CAD build for the part. Positions are in the model's coordinates, mm. Face numbers are marked on the shaded views. A direction names the side the tool comes from. Give positions to 0.01 mm unless a question says otherwise; leave off trailing zeros. Loops run counter-clockwise (first coordinate to the right, second up) from the corner with the lowest first, then second, coordinate; pieces in that order, holes last.
Item 1: Probe probe 1 along Y at (x, z) = (0, 6); probe 2 along Y at (x, z) = (0, -6.25); probe 3 along Y at (x, z) = (-18, 3.5). List the from-to ranges inside material, lowest first.
Item 2: Saw through at B-B on z = -10. Give the cut face in (x, y).
Item 3: Drop flat-ended pins along their axis: P1, Ø1.3, axis at y = 19, z = 0, coming from the +X side; P2, Ø3.5, axis at y = -18.5, z = 4.5, coming from the -X side; P3, Ø5, axis at x = 14, y = -3, coming from the -Z side; P4, Ø6, axis at x = -0.5, z = 5, coming from the +Y side. Give the stop position or say it passes through.
Item 4: Mould opens along X. For the marked faces 6, 7, 8 and 9 say: released by +X, released by -X, zero draft, split by the parting line, or undercut.
Item 5: Which spindle directions (+Z, -Z, +X, -X, +Y, -Y) get a long thin tool onto all of the face, cutting with end or side? Do the marked faces 1, 2, 3, 4 and 5. Say none if no direction does.
Item 6: Saw through at A-A on z = -5.75. Give the cut face in (x, y), plus the area to 3 significant figures.
Item 7: Saw through at C-C on x = -13.5. Give the cut face in (y, z).
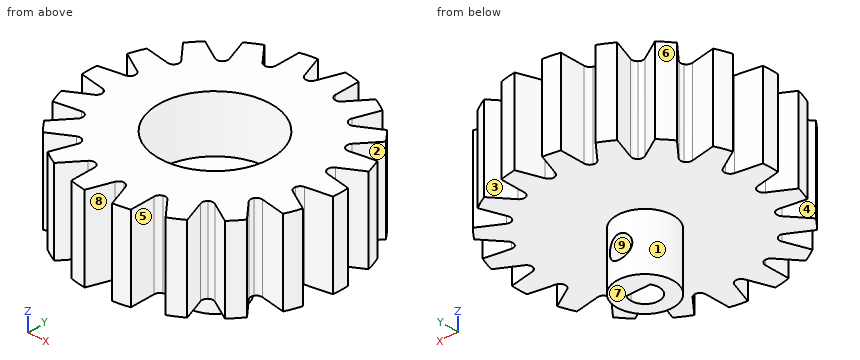
from build123d import *

# Parameters (mm, degrees)
F0_R            = 10
F0_R_2          = 5
F1_DEPTH        = 5
F2_DEPTH        = 15
F3_R            = 2
F4_DEPTH        = 8.6998377653
F0_R_3          = 22.5
F0_R_4          = 17.5
F5_DEPTH        = 5
F6_DEPTH        = 10
F8_DEPTH        = 25.0010001
F8_COPIES_COUNT = 18


# Not quite as in the source:
# - a feature of the source that left no trace in its solid (it failed there, or was rolled back) is left out
# - a pattern or mirror of a feature is missing from the dataset's text; its kind, count and spacing are read off the source's solid


with BuildPart() as f1:
    # F0 (on Top) → F1 (new body)
    with BuildSketch(Plane.XY):
        Circle(F0_R)
        Circle(F0_R_2, mode=Mode.SUBTRACT)
    extrude(amount=-F1_DEPTH)

    # F0 (on Top) → F2 (join)
    with BuildSketch(Plane.XY):
        Circle(F0_R_2)
        with BuildLine():
            ThreePointArc((2.1347076706, 1.3011622347), (2.4069450738, 0.6757332401), (2.5, 0))
            ThreePointArc((2.5, 0), (-0.6757332401, -2.4069450738), (-2.1347076706, 1.3011622347))
            ThreePointArc((-2.1347076706, 1.3011622347), (0, 2.5), (2.1347076706, 1.3011622347))
        make_face(mode=Mode.SUBTRACT)
        with BuildLine():
            Line((-2.1347076706, 1.3011622347), (2.1347076706, 1.3011622347))
            ThreePointArc((2.1347076706, 1.3011622347), (0, 2.5), (-2.1347076706, 1.3011622347))
        make_face()
    extrude(amount=-F2_DEPTH)

    # F3 (on face) → F4 (cut, through all)
    with BuildSketch(Plane.XZ.offset(-1.3011622347)):
        with Locations((0, -10)):
            Circle(F3_R)
    extrude(amount=-F4_DEPTH, mode=Mode.SUBTRACT)

    # F0 (on Top) → F5 (join)
    with BuildSketch(Plane.XY):
        Circle(F0_R_3)
        Circle(F0_R_4, mode=Mode.SUBTRACT)
        Circle(F0_R_4)
        Circle(F0_R, mode=Mode.SUBTRACT)
    extrude(amount=-F5_DEPTH)

    # F0 (on Top) → F6 (join)
    with BuildSketch(Plane.XY):
        Circle(F0_R_3)
        Circle(F0_R_4, mode=Mode.SUBTRACT)
        Circle(F0_R_4)
        Circle(F0_R, mode=Mode.SUBTRACT)
    extrude(amount=F6_DEPTH)

    # F7 (on face) → F8 (cut, through all)
    with BuildSketch(Plane.XY.offset(10)):
        with BuildLine():
            Line((0.9396926208, 18.1579798567), (2.470541887, 22.3639536483))
            ThreePointArc((2.470541887, 22.3639536483), (0, 22.5), (-2.470541887, 22.3639536483))
            Line((-2.470541887, 22.3639536483), (-0.9396926208, 18.1579798567))
            ThreePointArc((-0.9396926208, 18.1579798567), (-0.5735764364, 17.6808479557), (0, 17.5))
            ThreePointArc((0, 17.5), (0.5735764364, 17.6808479557), (0.9396926208, 18.1579798567))
        make_face()
    f8 = extrude(amount=-F8_DEPTH, mode=Mode.SUBTRACT)

    # F8_copies: F8 ×18 about axis
    f8_copies_axis = Axis((0, 0, 0), (0, 0, 1))
    for i in range(1, F8_COPIES_COUNT):
        add(f8.rotate(f8_copies_axis, i * 360 / F8_COPIES_COUNT), mode=Mode.SUBTRACT)


solid = f1.part
Results below:
1. probe 1: y = -17.5 to -10, 10 to 17.5
1. probe 2: y = -5 to -2.5, 1.3 to 5
1. probe 3: y = -13.5 to -13.16, -8.58 to -4.24, -2.24 to 2.24, 4.24 to 8.58, 13.16 to 13.5
2. outline: (-2.13, 1.3) - (-2, 1.3) - (-2, 4.58) arc R5 ccw (long way) to (2, 4.58) - (2, 1.3) - (2.13, 1.3) arc R2.5 cw (long way) to start
3. P1: stops at x = 12.48
3. P2: stops at x = -12.48
3. P3: stops at z = -5
3. P4: stops at y = 22.36
4. face 6: released by -X
4. face 7: zero draft
4. face 8: undercut
4. face 9: undercut
5. face 1: -Z
5. face 2: +Z, -Z, +X
5. face 3: +Z, -Z, +Y
5. face 4: +Z, -Z, -X
5. face 5: +Z, -Z, -Y
6. outline: circle Ø10 at (0, 0); hole (-2.13, 1.3) arc R2.5 ccw (long way) to (2.13, 1.3) - close
6. area: 62.5 mm2
7. outline: (-13.95, -5) - (13.95, -5) - (13.95, 10) - (-13.95, 10) - close
